Can you work these out from the drawing? Everything is in mm from the part's minimum corner. Coordinates: 2 decimals unless noted, no trailing zeros. Write each loop counter-clockwise with the first axis right and the second up, starting at its lowest first coordinate (ties: lowest second). Pieces come first, ordered by that corner, then holes.
(1) Imagine slicing it at A-A, the plane y = 4. List the corners of the cut face in (x, z) for me.
(2) Thinking about a two-plate mould opening in Y: for the marked faces 1, 2, 3 and 4, which applies, released by +Y, released by -Y, zero draft, split by the parting line, or undercut?
(3) Imagine slicing it at C-C, the plane y = 6.5. List the corners of the cut face in (x, z) for me.
(4) Please list where these lines run through material, in increasing order: probe 1 along X at (y, z) = (3, 3.5); probe 2 along X at (y, z) = (3.25, 2); probe 3 along Z at (x, y) = (1.5, 4.5).
(5) Imagine slicing it at B-B, the plane z = 5. List the corners of the cut face in (x, y) for me.
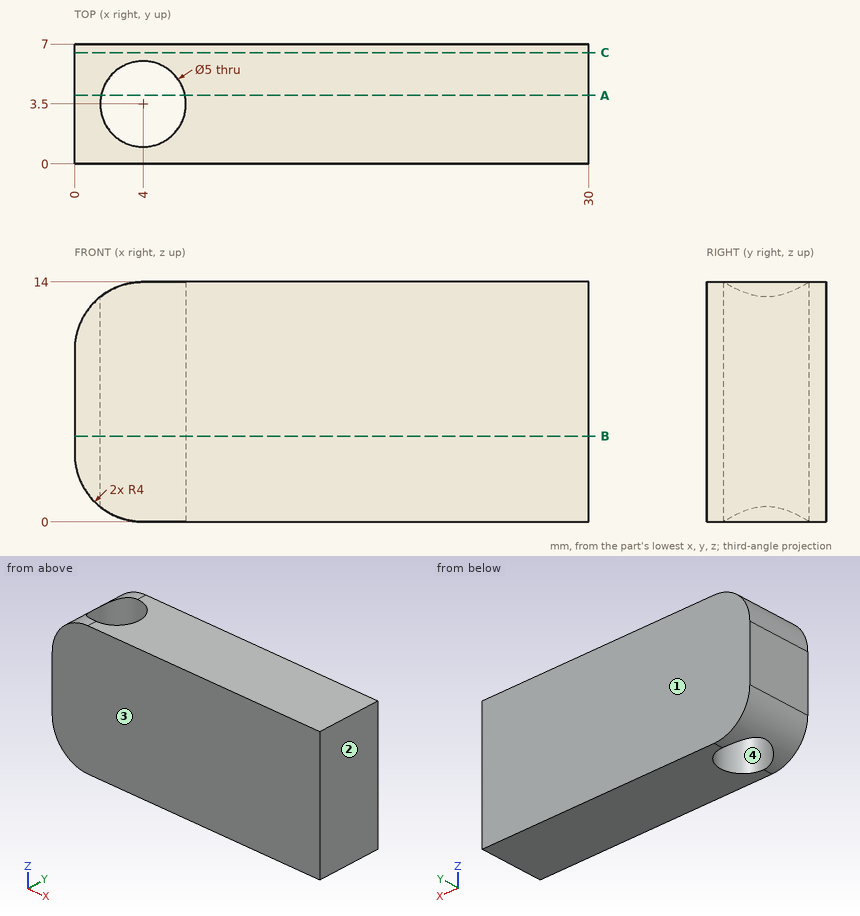
Recorded:
1. outline: (0, 4) arc R4 ccw to (1.55, 0.84) - (1.55, 13.16) arc R4 ccw to (0, 10) - close; (6.45, 0) - (30, 0) - (30, 14) - (6.45, 14) - close
2. face 1: released by +Y
2. face 2: zero draft
2. face 3: released by -Y
2. face 4: undercut
3. outline: (0, 4) arc R4 ccw to (4, 0) - (30, 0) - (30, 14) - (4, 14) arc R4 ccw to (0, 10) - close
4. probe 1: x = 0.03 to 1.55, 6.45 to 30
4. probe 2: x = 0.54 to 1.51, 6.49 to 30
4. probe 3: z = 0.88 to 13.12
5. outline: (0, 0) - (30, 0) - (30, 7) - (0, 7) - close; hole circle Ø5 at (4, 3.5)
